```python
from build123d import *

# Parameters (mm, degrees)
CIRCLE003_R                                  = 2
EXTRUDE087_DEPTH                             = 5
CIRCLE004_R                                  = 2
EXTRUDE088_DEPTH                             = 5
RECTANGLE026_W                               = 23
RECTANGLE026_H                               = 20
EXTRUDE019_DEPTH                             = 5
CHAMFER006_SIZE                              = 16
RECTANGLE028_AS_DRAWN_W                      = 22.6
RECTANGLE028_AS_DRAWN_H                      = 4
EXTRUDE033_DEPTH                             = 2.5
EXTRUDE033_ONTO_RECTANGLE028_ROLL_ANGLE      = 89.999906
EXTRUDE033_ONTO_RECTANGLE028_PITCH_ANGLE     = -44.999767
EXTRUDE033_ONTO_RECTANGLE028_PLACEMENT_ANGLE = 89.999906
RECTANGLE029_W                               = 24
RECTANGLE029_H                               = 4
EXTRUDE034_DEPTH                             = 2.5
RECTANGLE030_W                               = 4
RECTANGLE030_H                               = 4
EXTRUDE035_DEPTH                             = 2.5
RECTANGLE027_W                               = 17
RECTANGLE027_H                               = 20
EXTRUDE020_DEPTH                             = 5
RECTANGLE025_W                               = 23
RECTANGLE025_H                               = 60
EXTRUDE018_DEPTH                             = 5


with BuildPart() as extrude087:
    # Circle003 → Extrude087 (new body)
    with BuildSketch(Plane(origin=(-135, 30, 25), x_dir=(0, 1, 0), z_dir=(1, 0, 0))):
        Circle(CIRCLE003_R)
    extrude(amount=-EXTRUDE087_DEPTH)


with BuildPart() as extrude088:
    # Circle004 → Extrude088 (new body)
    with BuildSketch(Plane(origin=(-135, 30, 70), x_dir=(0, 1, 0), z_dir=(1, 0, 0))):
        Circle(CIRCLE004_R)
    extrude(amount=-EXTRUDE088_DEPTH)


with BuildPart() as chamfer006:
    # Rectangle026 → Extrude019 (new body)
    with BuildSketch(Plane(origin=(0, 17, 70), x_dir=(0, 1, 0), z_dir=(1, 0, 0))):
        with Locations((11.5, 10)):
            Rectangle(RECTANGLE026_W, RECTANGLE026_H)
    extrude(amount=EXTRUDE019_DEPTH)


with BuildPart() as chamfer006_1:
    # Extrude019 placement: moved
    add(chamfer006.part.moved(Location((0, -17, 0))))

    # Chamfer006
    chamfer006_edges = [chamfer006_1.edges().sort_by_distance(p)[0] for p in [
        (2.5, 0, 90),
    ]]
    chamfer(chamfer006_edges, length=CHAMFER006_SIZE)


with BuildPart() as chamfer006_2:
    # Chamfer006 placement: moved
    add(chamfer006_1.part.moved(Location((-140, 0, 0))))


with BuildPart() as extrude033:
    # Rectangle028 as drawn → Extrude033 (new)
    with BuildSketch(Plane.XY):
        with Locations((11.3, 2)):
            Rectangle(RECTANGLE028_AS_DRAWN_W, RECTANGLE028_AS_DRAWN_H)
    extrude(amount=EXTRUDE033_DEPTH)


with BuildPart() as extrude033_1:
    # Extrude033 onto Rectangle028 roll: moved
    add(extrude033.part.rotate(Axis((0, 0, 0), (1, 0, 0)), EXTRUDE033_ONTO_RECTANGLE028_ROLL_ANGLE))


with BuildPart() as extrude033_2:
    # Extrude033 onto Rectangle028 pitch: moved
    add(extrude033_1.part.rotate(Axis((0, 0, 0), (0, 1, 0)), EXTRUDE033_ONTO_RECTANGLE028_PITCH_ANGLE))


with BuildPart() as extrude033_3:
    # Extrude033 onto Rectangle028 placement: moved
    add(extrude033_2.part.moved(Location((5, 2.85, 71.15))).rotate(Axis((5, 2.85, 71.15), (0, 0, 1)), EXTRUDE033_ONTO_RECTANGLE028_PLACEMENT_ANGLE))


with BuildPart() as extrude033_4:
    # Extrude033 placement: moved
    add(extrude033_3.part.moved(Location((-147.5, 0, 0))))


with BuildPart() as extrude034:
    # Rectangle029 → Extrude034 (new body)
    with BuildSketch(Plane(origin=(5, 16, 86), x_dir=(0, 1, 0), z_dir=(1, 0, 0))):
        with Locations((12, 2)):
            Rectangle(RECTANGLE029_W, RECTANGLE029_H)
    extrude(amount=EXTRUDE034_DEPTH)


with BuildPart() as extrude034_1:
    # Extrude034 placement: moved
    add(extrude034.part.moved(Location((-147.5, 0, 0))))


with BuildPart() as extrude035:
    # Rectangle030 → Extrude035 (new body)
    with BuildSketch(Plane(origin=(5, 0, 70), x_dir=(0, 1, 0), z_dir=(1, 0, 0))):
        with Locations((2, 2)):
            Rectangle(RECTANGLE030_W, RECTANGLE030_H)
    extrude(amount=EXTRUDE035_DEPTH)


with BuildPart() as extrude035_1:
    # Extrude035 placement: moved
    add(extrude035.part.moved(Location((-147.5, 0, 0))))


with BuildPart() as fusion:
    # Rectangle027 → Extrude020 (new body)
    with BuildSketch(Plane(origin=(0, 0, 70), x_dir=(0, 1, 0), z_dir=(1, 0, 0))):
        with Locations((8.5, 10)):
            Rectangle(RECTANGLE027_W, RECTANGLE027_H)
    extrude(amount=EXTRUDE020_DEPTH)


with BuildPart() as fusion_1:
    # Extrude020 placement: moved
    add(fusion.part.moved(Location((-140, 23, 0))))

    # Fusion: union Chamfer006, Extrude033, Extrude034, Extrude035
    add(chamfer006_2.part)
    add(extrude033_4.part)
    add(extrude034_1.part)
    add(extrude035_1.part)


with BuildPart() as fusion_2:
    # Fusion placement: moved
    add(fusion_1.part.moved(Location((0, 0, -10))))


with BuildPart() as cut008:
    # Rectangle025 → Extrude018 (new body)
    with BuildSketch(Plane(origin=(0, 17, 10), x_dir=(0, 1, 0), z_dir=(1, 0, 0))):
        with Locations((11.5, 30)):
            Rectangle(RECTANGLE025_W, RECTANGLE025_H)
    extrude(amount=EXTRUDE018_DEPTH)


with BuildPart() as cut008_1:
    # Extrude018 placement: moved
    add(cut008.part.moved(Location((-140, 0, 0))))

    # Fusion002: union Fusion
    add(fusion_2.part)

    # Cut006: cut Extrude088
    add(extrude088.part, mode=Mode.SUBTRACT)

    # Cut008: cut Extrude087
    add(extrude087.part, mode=Mode.SUBTRACT)


solid = cut008_1.part
```
Model file for the job. Use its own axes, mm. A direction names the side the tool comes from. Coordinates: 2 decimals unless noted, no trailing zeros. Order: outer loops, then holes, each group sorted by start corner. A loop starts at its lowest first (then second) coordinate and runs counter-clockwise, first axis right, second up. Notation, with made-up numbers: (32.5, 1) -> (70.5, 1) arc R31 ccw to (70.5, 38) -> close; hole circle Ø5 at (-27, -1.75). An arc over 180 degrees is marked (long way). Return JSON: item names as keys, results as strings.
Item 1: Slice it at B-B (z = 25). Write the cut outline in (x, y), then the cut area to 3 significant figures.
Model answer:
{"outline": "(-140, 17) -> (-135, 17) -> (-135, 28) -> (-140, 28) -> close; (-140, 32) -> (-135, 32) -> (-135, 40) -> (-140, 40) -> close", "area": "95.0 mm²"}
Item 2: Wall check: line 1 along Z through (x, y) = (-138.7, 30); line 2 along Y through (x, z) = (-136.25, 55); line 3 along Z through (x, y) = (-141.25, 38.5). Give the ranges that are in metal, low to high. Write a range as from..to.
Model answer:
{"line 1": "z = 10..23, 27..68, 72..80", "line 2": "y = 17..40", "line 3": "z = 76..80"}
Item 3: Slice it at A-A (y = 30). Write the cut outline in (x, z), then the cut area to 3 significant figures.
Model answer:
{"outline": "(-142.5, 76) -> (-140, 76) -> (-140, 72) -> (-135, 72) -> (-135, 80) -> (-142.5, 80) -> close; (-140, 10) -> (-135, 10) -> (-135, 23) -> (-140, 23) -> close; (-140, 27) -> (-135, 27) -> (-135, 68) -> (-140, 68) -> close", "area": "320 mm²"}
Item 4: Pin check, flat tips, straight feed: P1, Ø3, axis at x = -139, z = 20.5, coming from the -Y side; P2, Ø2, axis at x = -140.5, y = 8, coming from the -Z side; P3, Ø1.2, axis at x = -141.5, z = 63, coming from the +Y side; P4, Ø5, axis at y = 30, z = 25, coming from the +X side. Stop position of each tip, or through.
Model answer:
{"P1": "stops at y = 17", "P2": "stops at z = 60", "P3": "stops at y = 5.3", "P4": "stops at x = -135"}
Item 5: Slice it at D-D (x = -137.75). Write the cut outline in (y, z).
Model answer:
{"outline": "(0, 60) -> (17, 60) -> (17, 10) -> (40, 10) -> (40, 80) -> (16, 80) -> (0, 64) -> close; hole circle Ø4 at (30, 25); hole circle Ø4 at (30, 70)"}
Item 6: 3-axis set-ups, long thin cutter, end or side, ignore diameter. For faces 4 (the face through (-141, 4, 61)), 5 (the face through (-138, 8, 60)), 6 (the face through (-138, 28, 10)): which of +Z, -Z, +X, -X, +Y, -Y reach the whole face in a straight line?
Model answer:
{"face 4": "-Z, -X, +Y", "face 5": "-Z, +X, -X, -Y", "face 6": "-Z, +X, -X, +Y, -Y"}
Item 7: Mould opens along Y. For faces 1 (the face through (-135, 24, 45)), 2 (the face through (-137.465, 31.847, 24.234)), 3 (the face through (-138, 40, 45)) say: pulls with the +Y half, pulls with the -Y half, needs draft (parallel to the pull), parting line crosses it, or undercut.
Model answer:
{"face 1": "needs draft", "face 2": "undercut", "face 3": "pulls with the +Y half"}
Item 8: Slice it at C-C (x = -141). Write the cut outline in (y, z).
Model answer:
{"outline": "(0, 60) -> (4, 60) -> (4, 62.3) -> (17.7, 76) -> (40, 76) -> (40, 80) -> (16, 80) -> (16, 79.96) -> (0.04, 64) -> (0, 64) -> close"}
